Design review of the part built by this model. Coordinates are the model's own, in mm. Face numbers are marked on the shaded views. A direction names the side the tool comes from. Coordinates: 2 decimals unless noted, no trailing zeros. Write each loop counter-clockwise with the first axis right and the second up, starting at its lowest first coordinate (ties: lowest second). Pieces come first, ordered by that corner, then holes.
Q1. Clearance check with flat-ended pins moving along their axes: pin 1 Ø4 at (x, z) = (-20, 7.52) entering from +Y; pin 2 Ø2 at (y, z) = (14.5, 7) entering from -X; pin 3 Ø9 at (x, y) = (-13, 26) entering from +Z. State where each tip first meets the part, or that it passes through.
Q2. To check wall thickness, follow probe 1 along X at (y, z) = (15, 11); probe 2 along Z at (x, y) = (-20, 3.7); probe 3 along Y at (x, z) = (-3, 14.25). State the ranges of each line that lie inside material, in increasing order.
Q3. Add section A-A, the plane y = 22. Give the boundary of the cut face in (x, z).
Q4. Machinability: for the marked faces 1, 2 and 3, which of the approach directions +Z, -Z, +X, -X, +Y, -Y give a long, thin tool a straight path to every point of the face, cutting with its end or side? Answer none if there is none.
Q5. The part is to be moulded in two halves that separate along X. For the marked faces 4, 5 and 6, say which applies: +X half, -X half, draft (parallel to the pull), parting line (faces both ways), or undercut.
Q6. Add section D-D, the plane x = 12.5. Give the boundary of the cut face in (y, z), plus the area to 3 significant figures.
Q7. Add section C-C, the plane y = 7. Give the boundary of the cut face in (x, z).
Q8. Add section B-B, the plane z = 18.5. Give the boundary of the cut face in (x, y), plus the area to 3 significant figures.
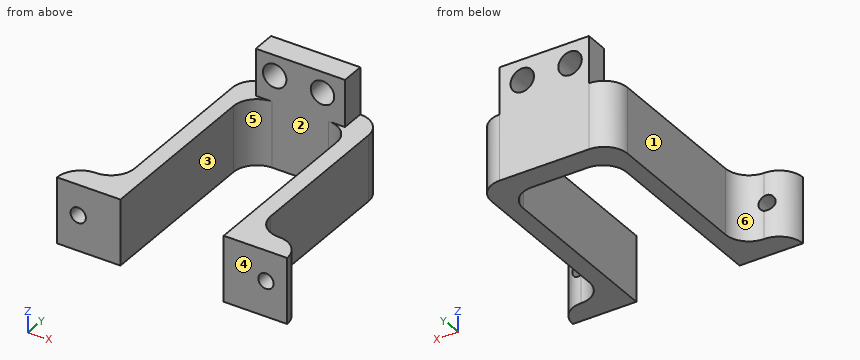
from build123d import *

# Parameters (mm, degrees)
BOSS_EXTRUDE1_DEPTH     = 14
FILLET1_R               = 5
FILLET2_R               = 5
CUT_EXTRUDE3_DEPTH      = 10
CUT_EXTRUDE3_DEPTH_BACK = 10
SKETCH2_R               = 1.636049027
SKETCH4_W               = 19
SKETCH4_H               = 5
BOSS_EXTRUDE2_DEPTH     = 10
SKETCH5_R               = 2.5
CUT_EXTRUDE4_DEPTH      = 10


with BuildPart() as part:
    # Sketch1 → Boss-Extrude1 (new body)
    with BuildSketch(Plane.XY):
        Polygon((-24.5, 0), (-24.5, 5), (-14.5, 5), (-14.5, 47), (14.5, 47), (14.5, 5), (24.5, 5), (24.5, 0), (11, 0), (11, 42), (-11, 42), (-11, 0), align=None)
    extrude(amount=BOSS_EXTRUDE1_DEPTH)

    # Fillet1
    fillet1_edges = [part.edges().sort_by_distance(p)[0] for p in [
        (-14.5, 47, 7),
        (14.5, 47, 7),
        (24.5, 5, 7),
        (-24.5, 5, 7),
        (14.5, 5, 7),
        (-14.5, 5, 7),
    ]]
    fillet(fillet1_edges, radius=FILLET1_R - 0.0001)  # a hair under: the kernel refuses the full size

    # Fillet2
    fillet2_edges = [part.edges().sort_by_distance(p)[0] for p in [
        (11, 42, 7),
        (-11, 42, 7),
    ]]
    fillet(fillet2_edges, radius=FILLET2_R)

    # Sketch2 → Cut-Extrude3 (cut, two sides: drawn at the far end of the back side and taken through both)
    with BuildSketch(Plane(origin=(0, 0, 0), x_dir=(1, 0, 0), z_dir=(0, 1, 0)).offset(-CUT_EXTRUDE3_DEPTH_BACK)):
        with Locations(Location((-20, -7.523321805, 0), (0, 0, 72.20487372))):
            Circle(SKETCH2_R)
        with Locations(Location((20, -7.523321805, 0), (0, 0, 107.795126278))):
            Circle(SKETCH2_R)
    extrude(amount=CUT_EXTRUDE3_DEPTH + CUT_EXTRUDE3_DEPTH_BACK, mode=Mode.SUBTRACT)

    # Sketch4 → Boss-Extrude2 (add)
    with BuildSketch(Plane.XY.offset(14)):
        with Locations((0, 44.5)):
            Rectangle(SKETCH4_W, SKETCH4_H)
    extrude(amount=BOSS_EXTRUDE2_DEPTH)

    # Sketch5 → Cut-Extrude4 (cut)
    with BuildSketch(Plane(origin=(0, 47, 0), x_dir=(1, 0, 0), z_dir=(0, 1, 0))):
        with Locations(Location((4.70575, -19.60149527, 0), (0, 0, 270))):
            Circle(SKETCH5_R)
        with Locations(Location((-5.477408827, -19.618067384, 0), (0, 0, 270))):
            Circle(SKETCH5_R)
    extrude(amount=-CUT_EXTRUDE4_DEPTH, mode=Mode.SUBTRACT)


solid = part.part
Here are the results:
1. pin 1: stops at y = 5.23
1. pin 2: stops at x = -14.5
1. pin 3: stops at z = 14
2. probe 1: x = -14.5 to -11, 11 to 14.5
2. probe 2: z = 0 to 5.89, 9.16 to 14
2. probe 3: y = 42 to 47
3. outline: (-14.5, 0) - (-11, 0) - (-11, 14) - (-14.5, 14) - close; (11, 0) - (14.5, 0) - (14.5, 14) - (11, 14) - close
4. face 1: +Z, -Z, -X, +Y
4. face 2: +Z, -Y
4. face 3: +Z, -Z, -Y
5. face 4: draft
5. face 5: undercut
5. face 6: -X half
6. outline: (0, 0) - (46, 0) - (46, 14) - (0, 14) - close
6. area: 644 mm2
7. outline: (-15.5, 0) - (-11, 0) - (-11, 14) - (-15.5, 14) - close; (11, 0) - (15.5, 0) - (15.5, 14) - (11, 14) - close
8. outline: (-9.5, 42) - (-7.71, 42) - (-7.71, 47) - (-9.5, 47) - close; (-3.24, 42) - (2.46, 42) - (2.46, 47) - (-3.24, 47) - close; (6.95, 42) - (9.5, 42) - (9.5, 47) - (6.95, 47) - close
8. area: 50.2 mm2
